```python
from build123d import *

# Parameters (mm, degrees)
F0_W     = 40
F0_H     = 40
F1_DEPTH = 25
F2_R     = 19.99999
F3_W     = 25
F3_H     = 20
F4_DEPTH = 20
F6_DEPTH = 15
F7_R     = 8
F8_DEPTH = 25
F9_SIZE  = 2
F10_W    = 3
F10_H    = 3


# Not quite as in the source:
# - a fillet or chamfer is up to 0.001 mm smaller than in the source, because OpenCascade refuses the exact size


with BuildPart() as f1:
    # F0 (on Top) → F1 (new body)
    with BuildSketch(Plane.XY):
        Rectangle(F0_W, F0_H)
    extrude(amount=F1_DEPTH)

    # F2 (radius 20 in the source; OpenCascade refuses exactly that, so slightly less here)
    f2_edges = [f1.edges().sort_by_distance(p)[0] for p in [
        (20, 20, 12.5),
        (-20, 20, 12.5),
    ]]
    fillet(f2_edges, radius=F2_R)

    # F3 (on face) → F4 (join)
    with BuildSketch(Plane.XZ.offset(20)):
        with Locations((0, 12.5)):
            Rectangle(F3_W, F3_H)
    extrude(amount=F4_DEPTH)

    # F5 (on face) → F6 (join)
    with BuildSketch(Plane.XZ.offset(40)):
        with BuildLine():
            ThreePointArc((0, 2.5), (7.0710678119, 5.4289321881), (10, 12.5))
            ThreePointArc((10, 12.5), (7.0710678119, 19.5710678119), (0, 22.5))
            ThreePointArc((0, 22.5), (-10, 12.5), (0, 2.5))
        make_face()
    extrude(amount=F6_DEPTH)

    # F7 (on face) → F8 (join)
    with BuildSketch(Plane.XY.offset(25)):
        Circle(F7_R)
    extrude(amount=F8_DEPTH)

    # F9
    f9_edges = [f1.edges().sort_by_distance(p)[0] for p in [
        (-8, 0, 50),
    ]]
    chamfer(f9_edges, length=F9_SIZE)

    # F10 (on Right) → F11 (revolve, cut)
    with BuildSketch(Plane.YZ):
        with Locations((-50.5, 22.5)):
            Rectangle(F10_W, F10_H)
    revolve(axis=Axis((0, -40, 12.5), (0, 1, 0)), mode=Mode.SUBTRACT)


solid = f1.part
```
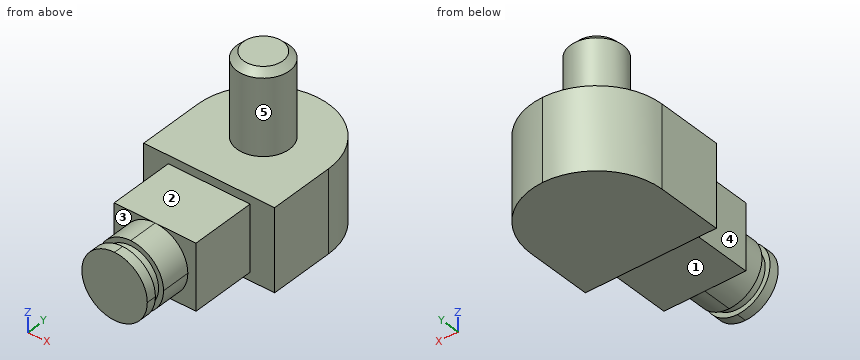
Could you check a few things on this model? Use its own coordinates, in mm. Face numbers are marked on the shaded views. A direction names the side the tool comes from. Give positions to 0.01 mm unless a question says otherwise; leave off trailing zeros. Write each loop counter-clockwise with the first axis right and the second up, starting at its lowest first coordinate (ties: lowest second). Pieces come first, ordered by that corner, then holes. Notation, with made-up numbers: (37.5, -37) - (71.5, -37) arc R33 cw to (71.5, -2) - close; hole circle Ø7 at (-36.75, -3.5). An arc over 180 degrees is marked (long way). One line per item, written item: value. Start each with the question number.
Item 1: Imagine slicing it at D-D, the plane y = -43. List the corners of the cut face in (x, z) for me.
Item 2: Which directions (+Z, -Z, +X, -X, +Y, -Y) give clear straight access to the entire face, cutting with the end or side of a thin tool? Please do the marked faces 1, 2, 3, 4 and 5.
Item 3: Please list where these lines run through material, in increasing order: line 1 (Z direction, x = -3, y = -16); line 2 (Z direction, x = -7, y = -36); line 3 (X direction, y = 0.5, z = 15.5). Write a range as from..to.
Item 4: I'm going to push flat-ended pins straight in: pin 1 (6 mm diameter, centred on y = -30.5, z = 9.5, fed in from -X); pin 2 (8 mm diameter, centred on x = -2.5, y = -41.5, fed in from -Z); pin 3 (10 mm diameter, centred on x = -5, y = -34, fed in from +Z); pin 4 (6 mm diameter, centred on x = -2, z = 9, fed in from +Y). Where does each tip first touch, or does it pass through?
Item 5: Imagine slicing it at C-C, the plane x = -13.5. List the corners of the cut face in (y, z) for me, and give its area (3 significant figures).
Item 6: Imagine slicing it at A-A, the plane y = -27. List the corners of the cut face in (x, z) for me.
Geometry says:
1. outline: circle Ø20 at (0, 12.5)
2. face 1: -Z, +X, -X, -Y
2. face 2: +Z, +X, -X, -Y
2. face 3: -X, -Y
2. face 4: +Z, -Z, -X, -Y
2. face 5: +Z
3. line 1: 0..25
3. line 2: 2.5..22.5
3. line 3: -19.99..19.99
4. pin 1: x = -12.5
4. pin 2: z = 2.5
4. pin 3: z = 22.5
4. pin 4: y = 20
5. outline: (-20, 0) - (14.76, 0) - (14.76, 25) - (-20, 25) - close
5. area: 869 mm^2
6. outline: (-12.5, 2.5) - (12.5, 2.5) - (12.5, 22.5) - (-12.5, 22.5) - close
